Verification items for the finished model (mm, model axes). A direction names the side the tool comes from. Give positions to 0.01 mm unless a question says otherwise; leave off trailing zeros. Loops run counter-clockwise (first coordinate to the right, second up) from the corner with the lowest first, then second, coordinate; pieces in that order, holes last. Notation, with made-up numbers: (-25, 61) -> (21, 61) arc R18 ccw to (21, 89) -> close; hole circle Ø7 at (63.25, 65.5). An arc over 180 degrees is marked (long way). Answer in a Markdown table with one row per item. Add a question column.
Q1. Section check C-C on y = 1.5. Enter the section's corners in (x, z) (3 decimals).
Q2. Gauge pin test, flat ends, axial feed: P1, Ø5, axis at x = -10, z = -10, coming from the -Y side; P2, Ø4, axis at x = 48.17, z = -10, coming from the -Y side; P3, Ø0.6, axis at y = 1, z = -27, coming from the +X side; P4, Ø1, axis at x = -7.5, y = 0.5, coming from the -Z side. Record the tip position at first contact, or that the pin passes through.
Q3. Section check A-A on z = -32. Enter the section's corners in (x, y), and give its area (3 significant figures).
Q4. Set-up check for faces 1 (the face through (19, 2, -20)), 2 (the face through (37.6, 1, -34)), 3 (the face through (36, 1, -27)), 4 (the face through (57.6, 1, -10)), 5 (the face through (-7, 1, -20)): record each of +Z, -Z, +X, -X, +Y, -Y from which the full face is reachable in a straight line by a thin tool's end or side.
Q5. Material ranges on probe 1 along X at (y, z) = (0.55, -10) (3 decimals); probe 2 along X at (y, z) = (1.4, -31.5); probe 3 along Z at (x, y) = (48.17, 1.3) (3 decimals), recorded low to high.
Q6. Section check B-B on x = -10. Enter the section's corners in (y, z) (3 decimals), and give its area (3 significant figures).
Q7. Section check D-D on x = 41. Enter the section's corners in (y, z), and give its area (3 significant figures).
Q8. Release check for a two-part mould opening along X. For faces 6 (the face through (50.133, 1.014, -9.186)), 7 (the face through (32.8, 1, -28)), 8 (the face through (56.17, 1.01, -18.5)), 9 (the face through (0.95, 1.01, -50.29)) record: pulls with the +X half, pulls with the -X half, needs draft (parallel to the pull), parting line crosses it, or undercut.
Autodesk Inventor part; units mm, degrees
ref_plane "YZ Plane" through (0, 0, 0) normal (1, 0, 0) x (0, 1, 0)
ref_plane "XZ Plane" through (0, 0, 0) normal (0, 1, 0) x (-1, 0, 0)
ref_plane "XY Plane" through (0, 0, 0) normal (0, 0, 1) x (1, 0, 0)
sketch "Sketch1" plane through (0, 0, 0) normal (0, 1, 0) x (-1, 0, 0)
  line L0 (0, 0) -> (-37.6, 0)
  line L1 (-37.6, -20) -> (-37.6, -51.2)
  line L2 (-37.6, -51.2) -> (0, -51.2)
  line L3 (0, -51.2) -> (0, -20)
  line L4 (-18.8, 0) -> (-1.65, 0)
  line L5 (-1.65, 0) -> (-23.35, 0)
  line L6 (-18.8, 0) -> (5.35, 0)
  line L7 (5.35, 0) -> (-25.85, 0)
  line L8 (-18.8, 0) -> (-3.2, 0)
  line L9 (-3.2, 0) -> (-34.4, 0)
  arc A0 (-32.8, -8.4) -> (-36, -8.4) centre (-34.4, -8.4) ccw
  arc A1 (-36, -46.5) -> (-32.8, -46.5) centre (-34.4, -46.5) ccw
  arc A2 (-1.6, -8.4) -> (-4.8, -8.4) centre (-3.2, -8.4) ccw
  arc A3 (-4.8, -46.5) -> (-1.6, -46.5) centre (-3.2, -46.5) ccw
  line L10 (0, 0) -> (0, -20)
  line L11 (0, -20) -> (20, -20)
  line L12 (20, -20) -> (20, 0)
  line L13 (20, 0) -> (0, 0)
  line L14 (-37.6, -20) -> (-57.6, -20)
  line L15 (-57.6, -20) -> (-57.6, 0)
  line L16 (-57.6, 0) -> (-37.6, 0)
  line L17 (-1.6, -46.5) -> (-1.6, -8.4)
  line L18 (-4.8, -8.4) -> (-4.8, -46.5)
  line L19 (-32.8, -46.5) -> (-32.8, -8.4)
  line L20 (-36, -8.4) -> (-36, -46.5)
  point P0 (5.35, 0)
  dimension "d0" = 37.6
  dimension "d1" = 51.2
  dimension "d41" = 15.6
  dimension "d42" = 31.2
  dimension "d50" = 3.2
  dimension "d56" = 3.2
  dimension "d57" = 3.2
  dimension "d63" = 3.2
  dimension "d67" = 8.4
  dimension "d77" = 8.4
  dimension "d81" = 20
  dimension "d82" = 20
  dimension "d83" = 20
extrude "Extrusion3" add sketch "Sketch1" along normal blind 2
fillet "Fillet2" radius 3.175 2 edges at (0, 1, -51.2) (37.6, 1, -51.2)
sketch "Sketch2" plane through (0, 2, 0) normal (0, 1, 0) x (1, 0, 0)
  circle A0 centre (-10, 10) radius 2.125
  line L0 (-20, 0) -> (57.6, 0)
  line L1 (38.17, 0) -> (48.17, 0)
  circle A1 centre (48.17, 10) radius 2.125
  point P0 (0, 0)
  dimension "d85" = 4.25
  dimension "d86" = 10
  dimension "d88" = 4.25
extrude "Extrusion4" cut sketch "Sketch2" against normal blind 2
fillet "Fillet3" radius 5 4 edges at (57.6, 1, -20) (57.6, 1, 0) (-20, 1, 0) (-20, 1, -20)
properties part number "Motor Attachment"
Taken from the geometry:
| question | item | result |
|---|---|---|
| 1 | outline | (-20, -15) arc R5 ccw to (-15, -20) -> (0, -20) -> (0, -48.025) arc R3.175 ccw to (3.175, -51.2) -> (34.425, -51.2) arc R3.175 ccw to (37.6, -48.025) -> (37.6, -20) -> (52.6, -20) arc R5 ccw to (57.6, -15) -> (57.6, -5) arc R5 ccw to (52.6, 0) -> (-15, 0) arc R5 ccw to (-20, -5) -> close; hole circle Ø4.25 at (-10, -10); hole (1.6, -46.5) arc R1.6 ccw to (4.8, -46.5) -> (4.8, -8.4) arc R1.6 ccw to (1.6, -8.4) -> close; hole (32.8, -46.5) arc R1.6 ccw to (36, -46.5) -> (36, -8.4) arc R1.6 ccw to (32.8, -8.4) -> close; hole circle Ø4.25 at (48.17, -10) |
| 2 | P1 | stops at y = 0 |
| 2 | P2 | passes through |
| 2 | P3 | stops at x = 37.6 |
| 2 | P4 | stops at z = -20 |
| 3 | outline | (0, 0) -> (1.6, 0) -> (1.6, 2) -> (0, 2) -> close; (4.8, 0) -> (32.8, 0) -> (32.8, 2) -> (4.8, 2) -> close; (36, 0) -> (37.6, 0) -> (37.6, 2) -> (36, 2) -> close |
| 3 | area | 62.4 mm² |
| 4 | face 1 | +Z, -Z, +X, -X, +Y |
| 4 | face 2 | -Z, +X, +Y, -Y |
| 4 | face 3 | +Y, -Y |
| 4 | face 4 | +Z, -Z, +X, +Y, -Y |
| 4 | face 5 | -Z, -X, +Y, -Y |
| 5 | probe 1 | x = -20 to -12.125, -7.875 to 1.6, 4.8 to 32.8, 36 to 46.045, 50.295 to 57.6 |
| 5 | probe 2 | x = 0 to 1.6, 4.8 to 32.8, 36 to 37.6 |
| 5 | probe 3 | z = -20 to -12.125, -7.875 to 0 |
| 6 | outline | (0, -20) -> (2, -20) -> (2, -12.125) -> (0, -12.125) -> close; (0, -7.875) -> (2, -7.875) -> (2, 0) -> (0, 0) -> close |
| 6 | area | 31.5 mm² |
| 7 | outline | (0, -20) -> (2, -20) -> (2, 0) -> (0, 0) -> close |
| 7 | area | 40.0 mm² |
| 8 | face 6 | undercut |
| 8 | face 7 | undercut |
| 8 | face 8 | pulls with the +X half |
| 8 | face 9 | pulls with the -X half |
